from build123d import *

# Parameters (mm, degrees)
REVOLVE1_ANGLE     = 360
SKETCH2_R          = 6.35
CUT_EXTRUDE1_DEPTH = 63.484
CIRPATTERN1_COUNT  = 5
CUT_EXTRUDE2_DEPTH = 7.62
CIRPATTERN2_COUNT  = 5
SKETCH5_R          = 1.1811
CUT_EXTRUDE3_DEPTH = 12.7
CIRPATTERN3_COUNT  = 6


with BuildPart() as part:
    # Sketch1 → Revolve1 (revolve, symmetric)
    with BuildSketch(Plane.XY) as revolve1_sk:
        Polygon((32.512, 43.053), (38.1, 43.053), (38.1, 0), (80.645, 0), (80.645, -16.383), (31.75, -16.383), (31.75, -62.484), (25.146, -62.484), (25.146, -49.577453141), (20.297971433, -41.110550681), (22.452839799, -41.110550681), (22.452839799, -6.400010137), (26.604598141, 18.108781172), (25.668560718, 18.108781172), (30.723038212, 27.881202719), (30.723038212, 29.21), (32.512, 29.21), align=None)
    revolve(axis=Axis((0, 66.608222053, 0), (0, -1, 0)), revolution_arc=REVOLVE1_ANGLE / 2)
    revolve(revolve1_sk.sketch, axis=Axis((0, 66.608222053, 0), (0, 1, 0)), revolution_arc=REVOLVE1_ANGLE / 2)

    # Sketch2 → Cut-Extrude1 (cut, through all)
    with BuildSketch(Plane(origin=(0, 0, 0), x_dir=(1, 0, 0), z_dir=(0, 1, 0))):
        with Locations((0, -57.15)):
            Circle(SKETCH2_R)
    cut_extrude1 = extrude(amount=-CUT_EXTRUDE1_DEPTH, mode=Mode.SUBTRACT)

    # CirPattern1: Cut-Extrude1 ×5 about axis
    cirpattern1_axis = Axis((0, 0, 0), (0, 1, 0))
    for i in range(1, CIRPATTERN1_COUNT):
        add(cut_extrude1.rotate(cirpattern1_axis, i * 360 / CIRPATTERN1_COUNT), mode=Mode.SUBTRACT)

    # Sketch3 → Cut-Extrude2 (cut)
    with BuildSketch(Plane(origin=(0, 0, 0), x_dir=(1, 0, 0), z_dir=(0, 1, 0))):
        with BuildLine():
            Line((-25.816115671, 58.929202602), (-17.918089551, 47.780088903))
            ThreePointArc((-17.918089551, 47.780088903), (0, 38.514784655), (17.918089551, 47.780088903))
            Line((17.918089551, 47.780088903), (25.816115671, 58.929202602))
            ThreePointArc((25.816115671, 58.929202602), (26.666104709, 64.585415867), (22.622433381, 68.630654062))
            ThreePointArc((22.622433381, 68.630654062), (0, 72.263), (-22.622433381, 68.630654062))
            ThreePointArc((-22.622433381, 68.630654062), (-26.666104709, 64.585415867), (-25.816115671, 58.929202602))
        make_face()
    cut_extrude2 = extrude(amount=-CUT_EXTRUDE2_DEPTH, mode=Mode.SUBTRACT)

    # CirPattern2: Cut-Extrude2 ×5 about axis
    cirpattern2_axis = Axis((0, 0, 0), (0, 1, 0))
    for i in range(1, CIRPATTERN2_COUNT):
        add(cut_extrude2.rotate(cirpattern2_axis, i * 360 / CIRPATTERN2_COUNT), mode=Mode.SUBTRACT)

    # Sketch5 → Cut-Extrude3 (cut)
    with BuildSketch(Plane.XZ.offset(62.484)):
        with Locations((0, 28.575)):
            Circle(SKETCH5_R)
    cut_extrude3 = extrude(amount=-CUT_EXTRUDE3_DEPTH, mode=Mode.SUBTRACT)

    # CirPattern3: Cut-Extrude3 ×6 about axis
    cirpattern3_axis = Axis((0, 0, 0), (0, 1, 0))
    for i in range(1, CIRPATTERN3_COUNT):
        add(cut_extrude3.rotate(cirpattern3_axis, i * 360 / CIRPATTERN3_COUNT), mode=Mode.SUBTRACT)


solid = part.part
For this review, take the finished solid that the model builds, in its own axes (mm). A direction names the side the tool comes from. Round coordinates to 2 decimals unless told otherwise and drop trailing zeros. Order: outer loops, then holes, each group sorted by start corner. A loop starts at its lowest first (then second) coordinate and runs counter-clockwise, first axis right, second up. Notation, with made-up numbers: (-26, 4.5) -> (-14, 4.5) arc R30 cw to (-14, 30.5) -> close; hole circle Ø10 at (74.25, 88.5). An arc over 180 degrees is marked (long way). Write item = value, one per line. Start each with the question number.
1) Take a section at C-C on y = -39. State the section outline as (x, z) points, plus the area to 3 significant figures.
2) Take a section at B-B on x = -3.5. Count the separate pieces of the cut face and the enclosed holes in it, plus the area to 3 significant figures.
3) Tool access review of faces 1 (the face through (59.56, -3.76, 36.66)), 2 (the face through (-60.674, -8.077, 18.267)), 3 (the face through (-5.45, -55.94, 24.55)): name each direction out of +Z, -Z, +X, -X, +Y, -Y from which nothing blocks a thin tool from reaching the whole face with its end or side.
4) Take a section at D-D on z = 45. State the section outline as (x, y) points, plus the area to 3 significant figures.
5) Take a section at A-A on z = -56.5. State the section outline as (x, y) points, plus the area to 3 significant figures.
6) Insertion check: pin 1 (10 mm diameter, centred on x = 0, z = 57.15, fed in from +Y); pin 2 (2 mm diameter, centred on x = 24.75, z = -14.29, fed in from +Y); pin 3 (21 mm diameter, centred on x = 34, z = 51, fed in from +Y); pin 4 (2 mm diameter, centred on x = -3, y = 21, fed in from -Z). Each pin has a flat end and moves straight along its axis. Give the tip position at first contact, or say it passes through.
7) To check wall thickness, follow line 1 (Z direction, x = 0, y = -56.5); line 2 (Z direction, x = 0, y = 28.45); line 3 (X direction, y = -7.5, z = 19). State the ranges of each line that lie inside material, in increasing order. Write a range as from..to.
Verdict:
q1.outline = circle Ø63.5 at (0, 0); hole circle Ø44.91 at (0, 0)
q1.area = 1,580 mm2
q2.separate_pieces = 3
q2.enclosed_holes = 0
q2.area = 3,110 mm2
q3.face_1 = +Y
q3.face_2 = +Y, -Y
q3.face_3 = -Y
q4.outline = (-66.92, -16.38) -> (66.92, -16.38) -> (66.92, 0) -> (56.54, 0) -> (56.54, -7.62) -> (13.94, -7.62) -> (13.94, 0) -> (-13.94, 0) -> (-13.94, -7.62) -> (-56.54, -7.62) -> (-56.54, 0) -> (-66.92, 0) -> close
q4.area = 1,540 mm2
q5.outline = (-57.54, -16.38) -> (57.54, -16.38) -> (57.54, 0) -> (24.1, 0) -> (24.1, -7.62) -> (-24.1, -7.62) -> (-24.1, 0) -> (-57.54, 0) -> close
q5.area = 1,520 mm2
q6.pin_1 = through
q6.pin_2 = 25.67
q6.pin_3 = -7.62
q6.pin_4 = -38.05
q7.line_1 = -31.75..-29.76, -27.39..-25.15, 25.15..27.39, 29.76..31.75
q7.line_2 = -38.1..-30.72, 30.72..38.1
q7.line_3 = -78.37..-60.56, -48.15..-11.96, 11.96..48.15, 60.56..78.37
